For this review, take the finished solid that the model builds, in its own axes (mm). Round coordinates to 2 decimals unless told otherwise and drop trailing zeros. Loops run counter-clockwise (first coordinate to the right, second up) from the corner with the lowest first, then second, coordinate; pieces in that order, holes last. Notation, with made-up numbers: (40.25, 4) -> (68.25, 4) arc R21 ccw to (68.25, 20) -> close; hole circle Ø6 at (38, 50). An arc over 180 degrees is marked (long way). One line per question, with ' | ' between items. Start each with the question number.
1. Draft analysis for pull direction X (two halves, no side actions). For faces 1 (the face through (-0.245, -1.103, -1.246)), 2 (the face through (0.01, -3.35, -0.1)), 3 (the face through (-2.9, -1.68, -0.1)), state which applies: pulls with the +X half, pulls with the -X half, needs draft (parallel to the pull), parting line crosses it, or undercut.
2. Consider section A-A (z = -1). Write out the cut boundary in (x, y) (3 decimals), and give its area (3 significant figures).
3. Wall thickness on line 1 along Y through (x, z) = (1, -1.85); line 2 along Y through (x, z) = (0.75, -1.9); line 3 along Y through (x, z) = (2.5, -1.2): over which ranges is each line inside the solid? List them lowest first.
4. For pin 1 Ø2.5 at (x, y) = (0, 0) entering from -Z, flat-tipped, find the tip position at first contact; note if it passes through.
```python
from build123d import *

# Parameters (mm, degrees)
BASENUT_START = -2.4892
BASENUTSKE_R  = 1.1303
BASENUT_DEPTH = 2.4892


with BuildPart() as part:
    # BaseNutSke → BaseNut (new body)
    with BuildSketch(Plane.XY.offset(BASENUT_START)):
        Polygon((3.175, 1.833087105), (3.175, -1.833087105), (0, -3.666174209), (-3.175, -1.833087105), (-3.175, 1.833087105), (0, 3.666174209), align=None)
        Circle(BASENUTSKE_R, mode=Mode.SUBTRACT)
    extrude(amount=BASENUT_DEPTH)

    # Sketch3 → Double-Chamfer (revolve, cut)
    with BuildSketch(Plane(origin=(0, 0, 0), x_dir=(0, 0, -1), z_dir=(1, 0, 0))):
        Polygon((2.4892, 3.175), (2.205620438, 3.666174209), (2.205620438, 16.366174209), (15.1892, 16.366174209), (15.1892, 3.175), align=None)
        Polygon((0.283579562, 16.366174209), (-12.7, 16.366174209), (-12.7, 3.175), (0, 3.175), (0.283579562, 3.666174209), align=None)
    revolve(axis=Axis((0, 0, 0), (0, 0, -1)), mode=Mode.SUBTRACT)

    # EndChamferSketch → EndChamfer (revolve, cut)
    with BuildSketch(Plane(origin=(0, 0, 0), x_dir=(0, 0, -1), z_dir=(1, 0, 0)), mode=Mode.PRIVATE) as endchamfer_sk:
        Polygon((2.4638, 1.4224), (2.238816316, 1.10109), (2.5146, 1.10109), (2.5146, 1.4224), align=None)
        Polygon((-0.0508, 1.4224), (0, 1.4224), (0.224983684, 1.10109), (-0.0508, 1.10109), align=None)
    revolve(endchamfer_sk.sketch.rotate(Axis((0, 0, -25.037505729), (0, 0, -1)), 90), axis=Axis((0, 0, -25.037505729), (0, 0, -1)), mode=Mode.SUBTRACT)


solid = part.part
```
Answer block:
1) face 1: undercut | face 2: parting line crosses it | face 3: pulls with the -X half
2) outline: (-3.175, -1.833) -> (0, -3.666) -> (3.175, -1.833) -> (3.175, 1.833) -> (0, 3.666) -> (-3.175, 1.833) -> close; hole circle Ø2.261 at (0, 0) | area: 30.9 mm2
3) line 1: y = -3.09 to -0.53, 0.53 to 3.09 | line 2: y = -3.23 to -0.85, 0.85 to 3.23 | line 3: y = -2.22 to 2.22
4) pin 1: stops at z = -2.34
